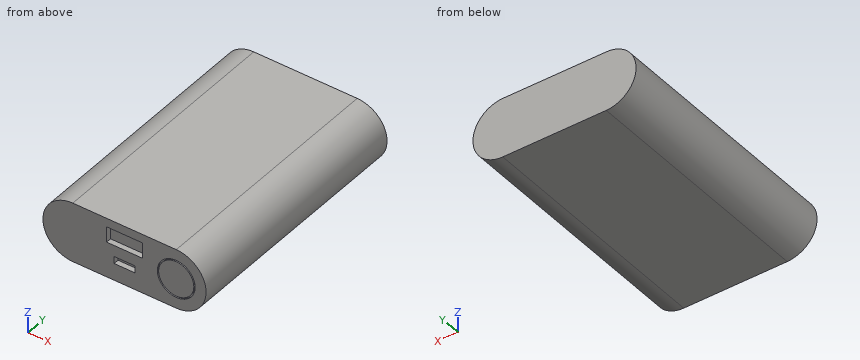
from build123d import *

# Parameters (mm, degrees)
F1_DEPTH = 91.3
F2_W     = 13.3
F2_H     = 5.8
F2_W_2   = 7.7
F2_H_2   = 2.66
F3_DEPTH = 2
F4_R     = 7
F4_R_2   = 6.5
F5_DEPTH = 0.5


with BuildPart() as f1:
    # F0 (on Front) → F1 (new body)
    with BuildSketch(Plane.XZ):
        with BuildLine():
            Line((49.35, 22.1), (11.05, 22.1))
            ThreePointArc((11.05, 22.1), (0, 11.05), (11.05, 0))
            Line((11.05, 0), (49.35, 0))
            ThreePointArc((49.35, 0), (60.4, 11.05), (49.35, 22.1))
        make_face()
    extrude(amount=F1_DEPTH)

    # F2 (on face) → F3 (cut)
    with BuildSketch(Plane.XZ.offset(91.3)):
        with Locations((30.2, 16)):
            Rectangle(F2_W, F2_H)
        with Locations((30.2, 7.63)):
            Rectangle(F2_W_2, F2_H_2)
    extrude(amount=-F3_DEPTH, mode=Mode.SUBTRACT)

    # F4 (on face) → F5 (cut)
    with BuildSketch(Plane.XZ.offset(91.3)):
        with Locations((49.35, 11.05)):
            Circle(F4_R)
        with Locations((49.35, 11.05)):
            Circle(F4_R_2, mode=Mode.SUBTRACT)
    extrude(amount=-F5_DEPTH, mode=Mode.SUBTRACT)


solid = f1.part
Geometry check sheet. Reference: the model listing, model coordinates, mm. Give positions to 0.01 mm unless a question says otherwise; leave off trailing zeros. Order: outer loops, then holes, each group sorted by start corner. A loop starts at its lowest first (then second) coordinate and runs counter-clockwise, first axis right, second up. Notation, with made-up numbers: M 89,77.25 L 116,77.25 A27 cw 116,107.25 Z; hole C 83,66.25 d10. An arc over 180 degrees is marked long. Use a Markdown table: item, result.
Item 1: Material ranges on line 1 along Z through (x, y) = (49, -91); line 2 along X through (y, z) = (-40.5, 2.5); line 3 along Y through (x, z) = (33.5, 8.75), recorded low to high.
Answers follow:
| item | result |
|---|---|
| line 1 | z = 0 to 4.06, 4.56 to 17.54, 18.04 to 22.1 |
| line 2 | x = 4.05 to 56.35 |
| line 3 | y = -89.3 to 0 |
Item 2: Section check B-B (z = 20.75). Record the cut outline in (x, y).
Answers follow:
| item | result |
|---|---|
| outline | M 5.76,-91.3 L 54.64,-91.3 L 54.64,0 L 5.76,0 Z |
Item 3: Section check A-A (y = -18). Record the cut outline in (x, z).
Answers follow:
| item | result |
|---|---|
| outline | M 11.05,0 L 49.35,0 A11.05 ccw 49.35,22.1 L 11.05,22.1 A11.05 ccw Z |
Item 4: Depth check by flat-ended pin: P1, Ø6, axis at y = -58.5, z = 18, coming from the -X side; P2, Ø4, axis at y = -45, z = 5.5, coming from the +X side; P3, Ø2, axis at y = -90, z = 7, coming from the +X side. Enter the tip coordinate at first touch or a pass-through.
Answers follow:
| item | result |
|---|---|
| P1 | stops at x = 0.73 |
| P2 | stops at x = 59.81 |
| P3 | stops at x = 59.97 |
